Work out the finished part from the listing and answer in its coordinate system (mm). A direction names the side the tool comes from. Give positions to 0.01 mm unless a question says otherwise; leave off trailing zeros. Write each loop counter-clockwise with the first axis right and the second up, starting at its lowest first coordinate (ties: lowest second). Pieces come first, ordered by that corner, then holes. Notation, with made-up numbers: (44.5, -13) -> (71.5, -13) arc R6 cw to (71.5, -4) -> close; hole circle Ø7 at (73.5, 23.25). An arc over 180 degrees is marked (long way). Use a Markdown table: item, result. Add a question column.
Q1. For a pull along Y with two mould halves and no side action, classify faces 1 (the face through (-15, 67, 3.8)), 2 (the face through (13.598, -64.196, 5.929)), 3 (the face through (-6, 61, 0)) as pulls with the +Y half, pulls with the -Y half, needs draft (parallel to the pull), parting line crosses it, or undercut.
Q2. For faces 4 (the face through (-49.757, 49.588, 1.927)), 5 (the face through (44.9, -44.9, 5.9)), determine the directions among +Z, -Z, +X, -X, +Y, -Y from which every point of the face is accessible in a straight line to the end or side of a thin tool.
Q3. Each of these flat-tipped pins is pushed along its axis until it touches: pin 1 Ø4 at (y, z) = (5, 3) entering from +X; pin 2 Ø2.5 at (x, y) = (15.5, 65) entering from +Z; pin 3 Ø3 at (y, z) = (-53, 1) entering from -X. Where does it stop, or does it pass through?
Q4. Section D-D, the plane y = 56 is taken. Give the vertices of the cut face in (x, z), plus the area to 3 significant figures.
Q5. Consider line 1 (Y direction, x = 39.5, z = 0.5); line 2 (X direction, y = 8.5, z = 2); line 3 (X direction, y = -17, z = 2). Determine where each line is inside the solid, lowest interval first.
Q6. Section A-A, the plane z = 2 is taken. State how many separate pieces and enclosed holes the cut face has, plus the area to 3 significant figures.
Q7. Section B-B, the plane y = 0 is taken. Give the vertices of the cut face in (x, z), plus the area to 3 significant figures.
from build123d import *

# Parameters (mm, degrees)
SKETCH1_R            = 75
BOSS_EXTRUDE1_DEPTH  = 8
M5_CLEARANCE_HOLE1_D = 5.5
CUT_EXTRUDE2_DEPTH   = 4.2
SKETCH11_R           = 45.85
CUT_EXTRUDE3_DEPTH   = 6
SKETCH12_R           = 60.7695
SKETCH12_R_2         = 53.6575
CUT_EXTRUDE4_DEPTH   = 4.1656


with BuildPart() as part:
    # Sketch1 → Boss-Extrude1 (new body)
    with BuildSketch(Plane.XY):
        Circle(SKETCH1_R)
    extrude(amount=BOSS_EXTRUDE1_DEPTH)

    # M5 Clearance Hole1 (through all)
    with Locations(Plane(origin=(0, 0, 0), x_dir=(-1, 0, 0), z_dir=(0, 0, -1))):
        with Locations((-17.470285544, -65.199993275), (-47.72970773, 47.72970773), (65.199993275, -17.470285544), (47.72970773, -47.72970773), (-65.199993275, 17.470285544), (-17.470285544, 65.199993275), (-65.199993275, -17.470285544), (-47.72970773, -47.72970773), (17.470285544, -65.199993275), (65.199993275, 17.470285544), (47.72970773, 47.72970773), (17.470285544, 65.199993275)):
            Hole(M5_CLEARANCE_HOLE1_D / 2)

    # Sketch6 → Cut-Extrude2 (cut)
    with BuildSketch(Plane(origin=(0, 0, 8), x_dir=(-1, 0, 0), z_dir=(0, 0, -1))):
        Polygon((-43.268287443, 46.534273767), (-44.463721406, 50.995694054), (-48.925141693, 52.191128017), (-52.191128017, 48.925141693), (-50.995694054, 44.463721406), (-46.534273767, 43.268287443), align=None)
        Polygon((-13.008865258, 66.395427237), (-16.274851582, 69.661413561), (-20.736271868, 68.465979598), (-21.931705831, 64.004559312), (-18.665719507, 60.738572988), (-14.204299221, 61.934006951), align=None)
        Polygon((21.931705831, 64.004559312), (20.736271868, 68.465979598), (16.274851582, 69.661413561), (13.008865258, 66.395427237), (14.204299221, 61.934006951), (18.665719507, 60.738572988), align=None)
        Polygon((50.995694054, 44.463721406), (52.191128017, 48.925141693), (48.925141693, 52.191128017), (44.463721406, 50.995694054), (43.268287443, 46.534273767), (46.534273767, 43.268287444), align=None)
        Polygon((66.395427237, 13.008865258), (69.661413561, 16.274851582), (68.465979598, 20.736271868), (64.004559312, 21.931705831), (60.738572988, 18.665719507), (61.934006951, 14.204299221), align=None)
        Polygon((64.004559312, -21.931705831), (68.465979598, -20.736271868), (69.661413561, -16.274851582), (66.395427237, -13.008865258), (61.934006951, -14.204299221), (60.738572988, -18.665719507), align=None)
        Polygon((44.463721406, -50.995694054), (48.925141693, -52.191128017), (52.191128017, -48.925141693), (50.995694054, -44.463721406), (46.534273767, -43.268287443), (43.268287444, -46.534273767), align=None)
        Polygon((13.008865258, -66.395427237), (16.274851582, -69.661413561), (20.736271868, -68.465979598), (21.931705831, -64.004559312), (18.665719507, -60.738572988), (14.204299221, -61.934006951), align=None)
        Polygon((-21.931705831, -64.004559312), (-20.736271868, -68.465979598), (-16.274851582, -69.661413561), (-13.008865258, -66.395427237), (-14.204299221, -61.934006951), (-18.665719507, -60.738572988), align=None)
        Polygon((-50.995694054, -44.463721406), (-52.191128017, -48.925141693), (-48.925141693, -52.191128017), (-44.463721406, -50.995694054), (-43.268287443, -46.534273767), (-46.534273767, -43.268287443), align=None)
        Polygon((-66.395427237, -13.008865258), (-69.661413561, -16.274851582), (-68.465979598, -20.736271868), (-64.004559312, -21.931705831), (-60.738572988, -18.665719507), (-61.934006951, -14.204299221), align=None)
        Polygon((-64.004559312, 21.931705831), (-68.465979598, 20.736271868), (-69.661413561, 16.274851582), (-66.395427237, 13.008865258), (-61.934006951, 14.204299221), (-60.738572988, 18.665719507), align=None)
    extrude(amount=CUT_EXTRUDE2_DEPTH, mode=Mode.SUBTRACT)

    # Sketch11 → Cut-Extrude3 (cut)
    with BuildSketch(Plane(origin=(0, 0, 0), x_dir=(-1, 0, 0), z_dir=(0, 0, -1))):
        Circle(SKETCH11_R)
    extrude(amount=-CUT_EXTRUDE3_DEPTH, mode=Mode.SUBTRACT)

    # Sketch12 → Cut-Extrude4 (cut)
    with BuildSketch(Plane(origin=(0, 0, 0), x_dir=(-1, 0, 0), z_dir=(0, 0, -1))):
        Circle(SKETCH12_R)
        Circle(SKETCH12_R_2, mode=Mode.SUBTRACT)
    extrude(amount=-CUT_EXTRUDE4_DEPTH, mode=Mode.SUBTRACT)


solid = part.part
Result set:
| question | item | result |
|---|---|---|
| 1 | face 1 | undercut |
| 1 | face 2 | undercut |
| 1 | face 3 | needs draft |
| 2 | face 4 | +Z, -Z |
| 2 | face 5 | +Z |
| 3 | pin 1 | stops at x = 74.94 |
| 3 | pin 2 | stops at z = 3.8 |
| 3 | pin 3 | stops at x = -54.52 |
| 4 | outline | (-49.89, 0) -> (-23.6, 0) -> (-23.6, 4.17) -> (23.6, 4.17) -> (23.6, 0) -> (49.89, 0) -> (49.89, 8) -> (-49.89, 8) -> close |
| 4 | area | 602 mm2 |
| 5 | line 1 | y = -63.76 to -46.18, -36.32 to -23.28, 23.28 to 36.32, 46.18 to 63.76 |
| 5 | line 2 | x = -74.52 to -60.17, -52.98 to -45.06, 45.06 to 52.98, 60.17 to 74.52 |
| 5 | line 3 | x = -73.05 to -67.91, -62.49 to -58.34, -50.89 to -42.58, 42.58 to 50.89, 58.34 to 62.49, 67.91 to 73.05 |
| 6 | separate pieces | 2 |
| 6 | enclosed holes | 14 |
| 6 | area | 8,230 mm2 |
| 7 | outline | (-75, 0) -> (-60.77, 0) -> (-60.77, 4.17) -> (-53.66, 4.17) -> (-53.66, 0) -> (-45.85, 0) -> (-45.85, 6) -> (45.85, 6) -> (45.85, 0) -> (53.66, 0) -> (53.66, 4.17) -> (60.77, 4.17) -> (60.77, 0) -> (75, 0) -> (75, 8) -> (-75, 8) -> close |
| 7 | area | 591 mm2 |
